from build123d import *

# Parameters (mm, degrees)
CROQUIS1_R              = 4
CROQUIS1_R_2            = 3
CROQUIS1_R_3            = 1.5
CROQUIS1_R_4            = 2
SALIENTE_EXTRUIR1_DEPTH = 5


with BuildPart() as part:
    # Croquis1 → Saliente-Extruir1 (new body)
    with BuildSketch(Plane.XY):
        with BuildLine():
            Line((102.068487159, -0.327277931), (102.068487159, -49.327277931))
            ThreePointArc((102.068487159, -49.327277931), (99.725341409, -54.98413218), (94.068487159, -57.327277931))
            Line((94.068487159, -57.327277931), (-89.931512841, -57.327277931))
            ThreePointArc((-89.931512841, -57.327277931), (-95.58836709, -54.98413218), (-97.931512841, -49.327277931))
            Line((-97.931512841, -49.327277931), (-97.931512841, -0.327277931))
            Line((-97.931512841, -0.327277931), (-97.931512841, 14.672722069))
            Line((-97.931512841, 14.672722069), (102.068487159, 14.672722069))
            Line((102.068487159, 14.672722069), (102.068487159, -0.327277931))
        make_face()
        with Locations((2.068487159, -27.327277931)):
            Circle(CROQUIS1_R, mode=Mode.SUBTRACT)
        with Locations((74.068487159, -19.577277931)):
            Circle(CROQUIS1_R_2, mode=Mode.SUBTRACT)
        with Locations((-69.931512841, -19.577277931)):
            Circle(CROQUIS1_R_2, mode=Mode.SUBTRACT)
        with Locations((74.068487159, -39.577277931)):
            Circle(CROQUIS1_R_3, mode=Mode.SUBTRACT)
        with Locations((54.068487159, -19.577277931)):
            Circle(CROQUIS1_R_3, mode=Mode.SUBTRACT)
        with Locations((94.068487159, -19.577277931)):
            Circle(CROQUIS1_R_3, mode=Mode.SUBTRACT)
        with Locations((-69.931512841, -39.577277931)):
            Circle(CROQUIS1_R_3, mode=Mode.SUBTRACT)
        with Locations((-89.931512841, -19.577277931)):
            Circle(CROQUIS1_R_3, mode=Mode.SUBTRACT)
        with Locations((-49.931512841, -19.577277931)):
            Circle(CROQUIS1_R_3, mode=Mode.SUBTRACT)
        with Locations((42.068487159, -45.327277931)):
            Circle(CROQUIS1_R_3, mode=Mode.SUBTRACT)
        with Locations((62.068487159, -45.327277931)):
            Circle(CROQUIS1_R_3, mode=Mode.SUBTRACT)
        with Locations((-57.931512841, -45.327277931)):
            Circle(CROQUIS1_R_3, mode=Mode.SUBTRACT)
        with Locations((-37.931512841, -45.327277931)):
            Circle(CROQUIS1_R_3, mode=Mode.SUBTRACT)
        with Locations((-12.931512841, -27.327277931)):
            Circle(CROQUIS1_R_3, mode=Mode.SUBTRACT)
        with Locations((17.068487159, -27.327277931)):
            Circle(CROQUIS1_R_3, mode=Mode.SUBTRACT)
        with Locations((2.068487159, -37.327277931)):
            Circle(CROQUIS1_R_3, mode=Mode.SUBTRACT)
        with Locations((-21.501512841, -3.757277931)):
            Circle(CROQUIS1_R_4, mode=Mode.SUBTRACT)
        with Locations((25.638487159, -3.757277931)):
            Circle(CROQUIS1_R_4, mode=Mode.SUBTRACT)
        with Locations((25.638487159, -50.897277931)):
            Circle(CROQUIS1_R_4, mode=Mode.SUBTRACT)
        with Locations((-21.501512841, -50.897277931)):
            Circle(CROQUIS1_R_4, mode=Mode.SUBTRACT)
        with Locations((32.068487159, -45.327277931)):
            Circle(CROQUIS1_R_3, mode=Mode.SUBTRACT)
        with Locations((-27.931512841, -45.327277931)):
            Circle(CROQUIS1_R_3, mode=Mode.SUBTRACT)
    extrude(amount=SALIENTE_EXTRUIR1_DEPTH)


solid = part.part
The listing builds one solid part. Answer for the finished solid, in the listing's coordinates (mm). Round coordinates to 2 decimals unless told otherwise and drop trailing zeros. Answer in a Markdown table with one row per item. Add a question column.
1) Consider line 1 along Y through (x, z) = (25, 4.15); line 2 along Y through (x, z) = (-23, 0.75); line 3 along X through (y, z) = (-37.5, 0.45). Determine where each line is inside the solid, lowest interval first. Write a range as from..to.
2) Determine the mould class of faces 1 (the face through (3, -21, 5)), 2 (the face through (99.79, -54.92, 2.46)), 3 (the face through (25, -49, 2)) for opening direction Y: pulls with the +Y half, pulls with the -Y half, needs draft (parallel to the pull), parting line crosses it, or undercut.
3) The part is cut by section A-A on z = 1.65. Count the separate pieces of the cut face and the enclosed holes in it, plus the area to 3 significant figures.
Findings below:
| question | item | result |
|---|---|---|
| 1 | line 1 | y = -57.33..-52.79, -49..-5.65, -1.86..14.67 |
| 1 | line 2 | y = -57.33..-52.22, -49.57..-5.08, -2.43..14.67 |
| 1 | line 3 | x = -97.93..0.58, 3.56..102.07 |
| 2 | face 1 | needs draft |
| 2 | face 2 | pulls with the -Y half |
| 2 | face 3 | undercut |
| 3 | separate pieces | 1 |
| 3 | enclosed holes | 22 |
| 3 | area | 14,100 mm² |
